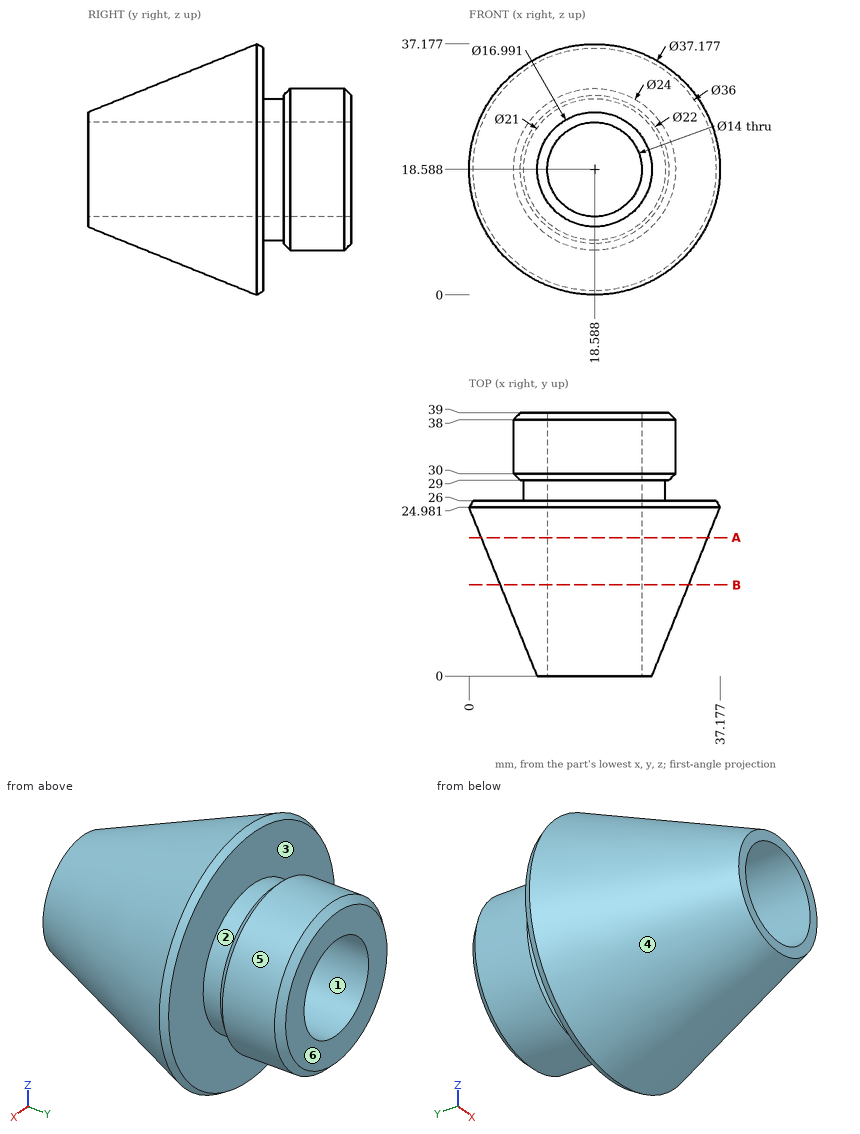
Input: dimensioned drawing with shaded views. Units: mm. Origin: part minimum x, y, z. A direction names the side the tool comes from. Give positions to 0.01 mm unless a question says otherwise; leave off trailing zeros. Loops run counter-clockwise (first coordinate to the right, second up) from the corner with the lowest first, then second, coordinate; pieces in that order, holes last. Notation, with made-up numbers: (-34.5, -28) -> (24.5, -28) arc R30 ccw to (24.5, 1) -> close; hole circle Ø7 at (-29.75, 60). An arc over 180 degrees is marked (long way). Use a Markdown table: item, result. Add a question column.
1) Section query B-B, the plane y = 13.5. Return the cut outline in (x, z), then the cut area to 3 significant figures.
2) Pull-direction query (Y, two-part tool) for the marked faces 3, 4, 5 and 6; classes: +Y half, -Y half, draft (parallel to the pull), parting line (faces both ways), or undercut.
3) First-contact query: pin 1 (4 mm diameter, centred on y = 24.5, z = 20, fed in from +X); pin 2 (8.5 mm diameter, centred on x = 18.59, z = 18.59, fed in from -Y); pin 3 (8 mm diameter, centred on y = 22, z = 12, fed in from +X); pin 4 (4 mm diameter, centred on x = 28, y = 10.5, fed in from -Z). Flat tips, straight axial feed; report the tip coordinate or a pass-through.
4) Reachability of the marked faces 1 and 2 from +Z, -Z, +X, -X, +Y, -Y: full face, straight path, thin tool, end or side. Return the list, or none.
5) Line query: line 1 along Z through (x, y) = (21, 28); line 2 along Z through (x, y) = (20, 32) (1 decimal); line 3 along Y through (x, z) = (7, 21) (1 decimal). Output: solid intervals per line, ascending. Write a range as [from, to].
6) Section query A-A, the plane y = 20.5. Return the cut outline in (x, z) (1 decimal).
Numbers:
| question | item | result |
|---|---|---|
| 1 | outline | circle Ø27.9 at (18.59, 18.59); hole circle Ø14 at (18.59, 18.59) |
| 1 | area | 457 mm2 |
| 2 | face 3 | undercut |
| 2 | face 4 | -Y half |
| 2 | face 5 | draft |
| 2 | face 6 | +Y half |
| 3 | pin 1 | stops at x = 37.18 |
| 3 | pin 2 | passes through |
| 3 | pin 3 | stops at x = 36.76 |
| 3 | pin 4 | stops at z = 7.92 |
| 4 | face 1 | +Y, -Y |
| 4 | face 2 | none |
| 5 | line 1 | z = [8.37, 12.02], [25.16, 28.81] |
| 5 | line 2 | z = [6.7, 11.7], [25.4, 30.5] |
| 5 | line 3 | y = [8.3, 26], [29.8, 38.2] |
| 6 | outline | circle Ø33.6 at (18.6, 18.6); hole circle Ø14 at (18.6, 18.6) |
